For this review, use the dimensioned drawing (mm, ordinates from the lowest corner) and the shaded views. Round coordinates to 2 decimals unless told otherwise and drop trailing zeros. Order: outer loops, then holes, each group sorted by start corner. A loop starts at its lowest first (then second) coordinate and runs counter-clockwise, first axis right, second up. Notation, with made-up numbers: M 53,49.25 L 112,49.25 A12 ccw 112,72.25 Z; hole C 51.5,64 d4. An arc over 180 degrees is marked long. One line per item, written item: value. Start each with the question number.
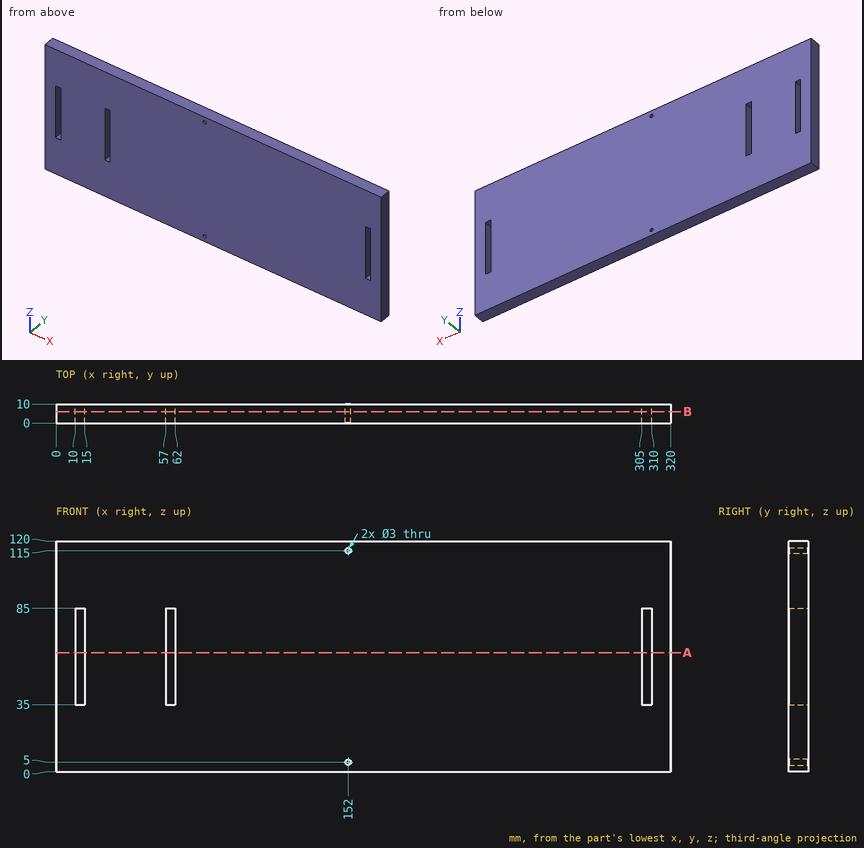
Item 1: Consider section A-A, the plane z = 62. Give the boundary of the cut face in (x, y), then the cut area to 3 significant figures.
Item 2: Wall thickness on L1, parallel to X at y = 8.75, z = 68; L2, parallel to Z at x = 152, y = 6.75; L3, parallel to X at y = 6.75, z = 5: over which ranges is each line inside the solid? List them lowest first.
Item 3: Consider section B-B, the plane y = 6. Give the boundary of the cut face in (x, z), then the cut area to 3 significant figures.
Computed:
1. outline: M 0,0 L 10,0 L 10,10 L 0,10 Z; M 15,0 L 57,0 L 57,10 L 15,10 Z; M 62,0 L 305,0 L 305,10 L 62,10 Z; M 310,0 L 320,0 L 320,10 L 310,10 Z
1. area: 3,050 mm^2
2. L1: x = 0 to 10, 15 to 57, 62 to 305, 310 to 320
2. L2: z = 0 to 3.5, 6.5 to 113.5, 116.5 to 120
2. L3: x = 0 to 150.5, 153.5 to 320
3. outline: M 0,0 L 320,0 L 320,120 L 0,120 Z; hole M 10,35 L 15,35 L 15,85 L 10,85 Z; hole M 57,35 L 62,35 L 62,85 L 57,85 Z; hole C 152,5 d3; hole C 152,115 d3; hole M 305,35 L 310,35 L 310,85 L 305,85 Z
3. area: 37,600 mm^2
